Here's how the part is built. I have some questions about the finished solid (model axes, mm). Face numbers are marked on the shaded views. A direction names the side the tool comes from. Coordinates: 2 decimals unless noted, no trailing zeros. Write each loop counter-clockwise with the first axis right and the second up, starting at its lowest first coordinate (ties: lowest second). Pieces come first, ordered by that corner, then holes.
(1) Imagine slicing it at B-B, the plane x = 11. List the corners of the cut face in (y, z) for me.
(2) Thinking about a two-plate mould opening in X: for the marked faces 3, 4 and 5, which applies, released by +X, released by -X, zero draft, split by the parting line, or undercut?
(3) Please list where these lines run through material, in increasing order: probe 1 along X at (y, z) = (-92.5, 39); probe 2 along Y at (x, z) = (-51, 20); probe 3 along Z at (x, y) = (30.5, -72.5).
(4) Imagine slicing it at D-D, the plane z = 20. List the corners of the cut face in (x, y) for me, plus the area to 3 significant figures.
(5) For pin 1 Ø23 at (x, z) = (9.93, 24.34) entering from -Y; pin 2 Ø1 at (x, y) = (0, -37) entering from -Z, each with a flat end and sliding along its axis, tell me the tip position at first contact or that it passes through.
(6) Which directions (+Z, -Z, +X, -X, +Y, -Y) give clear straight access to the entire face, cutting with the end or side of a thin tool? Please do the marked faces 1 and 2.
(7) Imagine slicing it at A-A, the plane y = -15. List the corners of the cut face in (x, z) for me.
(8) Imagine slicing it at C-C, the plane z = 95. List the corners of the cut face in (x, y) for me.
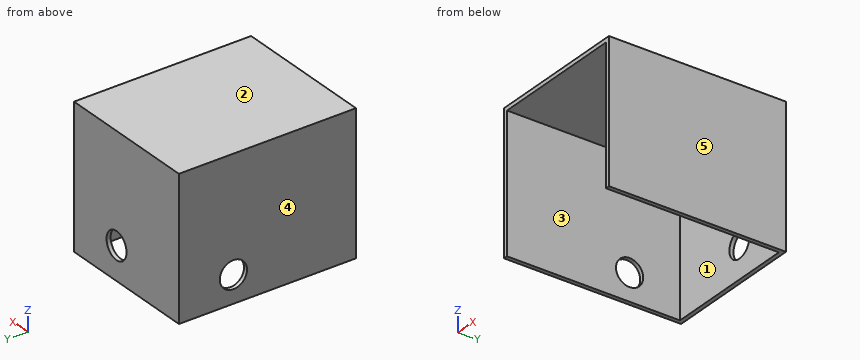
Autodesk Inventor part; units mm, degrees
ref_plane "YZ Plane" through (0, 0, 0) normal (1, 0, 0) x (0, 1, 0)
ref_plane "XZ Plane" through (0, 0, 0) normal (0, 1, 0) x (-1, 0, 0)
ref_plane "XY Plane" through (0, 0, 0) normal (0, 0, 1) x (1, 0, 0)
sketch "Sketch1" plane through (0, 0, 0) normal (0, 0, 1) x (1, 0, 0)
  line L0 (52.4625, 25) -> (-52.4625, 25)
  line L1 (-52.4625, 25) -> (-52.4625, -105)
  line L2 (52.4625, -105) -> (52.4625, 25)
  line L3 (-96.7125, -125) -> (96.7125, -125)
  line L4 (55.4625, -110) -> (55.4625, -50)
  line L5 (-55.4625, -50) -> (-55.4625, -110)
  line L6 (52.4625, -105) -> (49.4625, -105)
  line L7 (49.4625, -105) -> (49.4625, 22)
  line L8 (49.4625, 25) -> (52.4625, 25)
  line L9 (52.4625, 25) -> (52.4625, -105)
  line L10 (-52.4625, -105) -> (-49.4625, -105)
  line L11 (-49.4625, -105) -> (-49.4625, 22)
  line L12 (-49.4625, 25) -> (-52.4625, 25)
  line L13 (-52.4625, 25) -> (-52.4625, -105)
  line L14 (49.4625, 25) -> (-49.4625, 25)
  line L15 (-49.4625, 22) -> (49.4625, 22)
  line L16 (-52.4625, -105) -> (-49.4625, -105)
  line L17 (49.4625, -105) -> (52.4625, -105)
  point P0 (0, 0)
  point P1 (50.9625, -105)
  dimension "d7" = 127
  dimension "d8" = 20
  dimension "d9" = 3
  dimension "d10" = 3
  dimension "d11" = 98.925
  dimension "d12" = 3
  dimension "d13" = 3
extrude "Extrusion1" add sketch "Sketch1" along normal blind 100
sketch "Sketch2" plane through (0, 0, 100) normal (0, 0, 1) x (1, 0, 0)
  line L0 (52.4625, -105) -> (52.4625, 25)
  line L1 (-52.4625, 25) -> (-52.4625, -105)
  line L2 (52.4625, 25) -> (-52.4625, 25)
  line L3 (-52.4625, 25) -> (-52.4625, -105)
  line L4 (-52.4625, -105) -> (52.4625, -105)
  line L5 (52.4625, -105) -> (52.4625, 25)
  point P0 (0, 0)
extrude "Extrusion2" add sketch "Sketch2" along normal blind 3
sketch "Sketch3" plane through (-52.4625, -105, 0) normal (-1, 0, 0) x (0, 0, 1)
  circle A0 centre (20, 90) radius 10
  line L0 (0, 130) -> (0, 0)
  line L1 (0, 130) -> (103, 130)
  point P0 (0, 105)
  dimension "d18" = 20
  dimension "d19" = 20
  dimension "d20" = 40
extrude "Extrusion3" cut sketch "Sketch3" against normal blind 3
sketch "Sketch4" plane through (-49.4625, 22, 0) normal (0, -1, 0) x (1, 0, 0)
  circle A0 centre (59.3936, 24.3432) radius 10
  point P0 (49.4625, 0)
  dimension "d23" = 20
extrude "Extrusion4" cut sketch "Sketch4" against normal blind 3
properties part number "HANG"
Recorded:
1. outline: (-105, 100) - (22, 100) - (22, 34.29) - (25, 34.29) - (25, 103) - (-105, 103) - close; (22, 0) - (25, 0) - (25, 14.4) - (22, 14.4) - close
2. face 3: undercut
2. face 4: released by -X
2. face 5: released by +X
3. probe 1: x = -52.46 to -49.46, 49.46 to 52.46
3. probe 2: y = -105 to -25, -5 to 25
3. probe 3: z = 100 to 103
4. outline: (-52.46, -105) - (-49.46, -105) - (-49.46, -25) - (-52.46, -25) - close; (-52.46, -5) - (-49.46, -5) - (-49.46, 22) - (0.92, 22) - (0.92, 25) - (-52.46, 25) - close; (18.94, 22) - (49.46, 22) - (49.46, -105) - (52.46, -105) - (52.46, 25) - (18.94, 25) - close
4. area: 963 mm2
5. pin 1: stops at y = 22
5. pin 2: stops at z = 100
6. face 1: -Z, -Y
6. face 2: +Z, +X, -X, +Y, -Y
7. outline: (-52.46, 0) - (-49.46, 0) - (-49.46, 10) - (-52.46, 10) - close; (-52.46, 30) - (-49.46, 30) - (-49.46, 100) - (49.46, 100) - (49.46, 0) - (52.46, 0) - (52.46, 103) - (-52.46, 103) - close
8. outline: (-52.46, -105) - (-49.46, -105) - (-49.46, 22) - (49.46, 22) - (49.46, -105) - (52.46, -105) - (52.46, 25) - (-52.46, 25) - close
